```python
from build123d import *

# Parameters (mm, degrees)
F0_W     = 838.2
F0_H     = 508
F0_W_2   = 685.8
F0_H_2   = 355.6
F1_DEPTH = 254
F2_DEPTH = 279.4
F3_T     = -0.254


with BuildPart() as f1:
    # F0 (on Top) → F1 (new body)
    with BuildSketch(Plane.XY):
        with Locations((-259.4876274824, 118.1668707132)):
            Rectangle(F0_W, F0_H)
        with Locations((-259.4876274824, 118.1668707132)):
            Rectangle(F0_W_2, F0_H_2, mode=Mode.SUBTRACT)
        with Locations((-259.4876274824, 118.1668707132)):
            Rectangle(F0_W_2, F0_H_2)
    extrude(amount=F1_DEPTH)

    # F0 (on Top) → F2 (join)
    with BuildSketch(Plane.XY):
        with Locations((-259.4876274824, 118.1668707132)):
            Rectangle(F0_W_2, F0_H_2)
    extrude(amount=F2_DEPTH)

    # F3
    f3_openings = [f1.faces().sort_by_distance(p)[0] for p in [
        (-259.487627, 118.166871, 0),
    ]]
    offset(amount=F3_T, openings=f3_openings, kind=Kind.INTERSECTION)


solid = f1.part
```
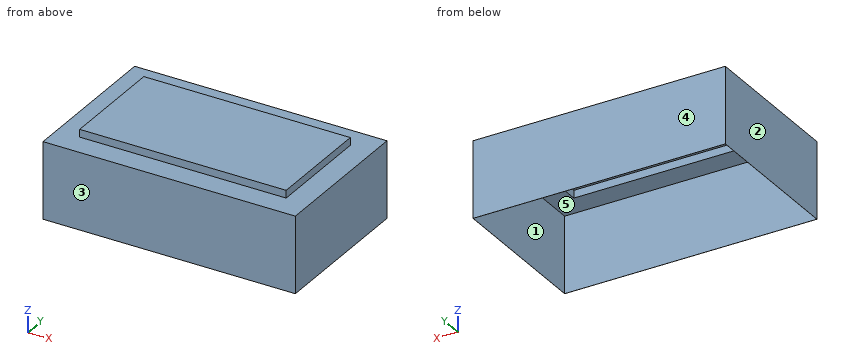
Here's how the part is built. I have some questions about the finished solid (model axes, mm). Face numbers are marked on the shaded views. A direction names the side the tool comes from. Give positions to 0.01 mm unless a question says otherwise; leave off trailing zeros. Order: outer loops, then holes, each group sorted by start corner. A loop starts at its lowest first (then second) coordinate and runs counter-clockwise, first axis right, second up. Notation, with made-up numbers: (67, 64) - (100, 64) arc R10 cw to (100, 72) - close; hole circle Ø10 at (-23, 35). An arc over 180 degrees is marked (long way). Answer as a JSON object with one key per item and string values. Group by question number.
Item 1: If we section it at D-D on y = 323.5: Please give me the cut outline in (x, z).
Item 2: If we section it at B-B on z = 112: Please give me the cut outline in (x, y), and give its area (3 significant figures).
Item 3: Please list where these lines run through material, in increasing order: probe 1 along X at (y, z) = (132, 53); probe 2 along Y at (x, z) = (108.5, 155); probe 3 along Y at (x, z) = (-382.5, 255).
Item 4: If we mould it in two halves opening along X, with no side actions, what happens to the marked faces 1, 2 and 3? For each: pulls with the +X half, pulls with the -X half, needs draft (parallel to the pull), parting line crosses it, or undercut.
Item 5: If we section it at C-C on x = -257: Please give me the cut outline in (y, z), and give its area (3 significant figures).
Item 6: If we section it at A-A on y = 235.5: Please give me the cut outline in (x, z), and give its area (3 significant figures).
Item 7: Which directions (+Z, -Z, +X, -X, +Y, -Y) give clear straight access to the entire face, cutting with the end or side of a thin tool? Please do the marked faces 4 and 5.
Item 8: For P1, Ø12.5, axis at y = 165.5, z = 272.5, coming from the +X side; P2, Ø7.5, axis at y = 80.5, z = 266, coming from the -X side; P3, Ø1.5, axis at x = -423.5, y = 106, coming from the -Z side, each with a flat end and sliding along its axis, tell me the tip position at first contact or that it passes through.
Result set:
{
 "1": {"outline": "(-678.59, 0) - (-678.33, 0) - (-678.33, 253.75) - (159.36, 253.75) - (159.36, 0) - (159.61, 0) - (159.61, 254) - (-678.59, 254) - close"},
 "2": {"outline": "(-678.59, -135.83) - (159.61, -135.83) - (159.61, 372.17) - (-678.59, 372.17) - close; hole (-678.33, -135.58) - (159.36, -135.58) - (159.36, 371.91) - (-678.33, 371.91) - close", "area": "684 mm²"},
 "3": {"probe 1": "-678.59 to -678.33, 159.36 to 159.61", "probe 2": "-135.83 to -135.58, 371.91 to 372.17", "probe 3": "-59.63 to -59.38, 295.71 to 295.97"},
 "4": {"face 1": "undercut", "face 2": "pulls with the -X half", "face 3": "needs draft"},
 "5": {"outline": "(-135.83, 0) - (-135.58, 0) - (-135.58, 253.75) - (-59.38, 253.75) - (-59.38, 279.15) - (295.71, 279.15) - (295.71, 253.75) - (371.91, 253.75) - (371.91, 0) - (372.17, 0) - (372.17, 254) - (295.97, 254) - (295.97, 279.4) - (-59.63, 279.4) - (-59.63, 254) - (-135.83, 254) - close", "area": "271 mm²"},
 "6": {"outline": "(-678.59, 0) - (-678.33, 0) - (-678.33, 253.75) - (-602.13, 253.75) - (-602.13, 279.15) - (83.16, 279.15) - (83.16, 253.75) - (159.36, 253.75) - (159.36, 0) - (159.61, 0) - (159.61, 254) - (83.41, 254) - (83.41, 279.4) - (-602.39, 279.4) - (-602.39, 254) - (-678.59, 254) - close", "area": "355 mm²"},
 "7": {"face 4": "+Z, -Z, +X, -X, +Y", "face 5": "-Z"},
 "8": {"P1": "x = 83.41", "P2": "x = -602.39", "P3": "z = 279.15"}
}
